Work out the finished part from the listing and answer in its coordinate system (mm). Face numbers are marked on the shaded views. A direction names the side the tool comes from. Give positions to 0.01 mm unless a question says otherwise; leave off trailing zeros. Loops run counter-clockwise (first coordinate to the right, second up) from the corner with the lowest first, then second, coordinate; pieces in that order, holes last.
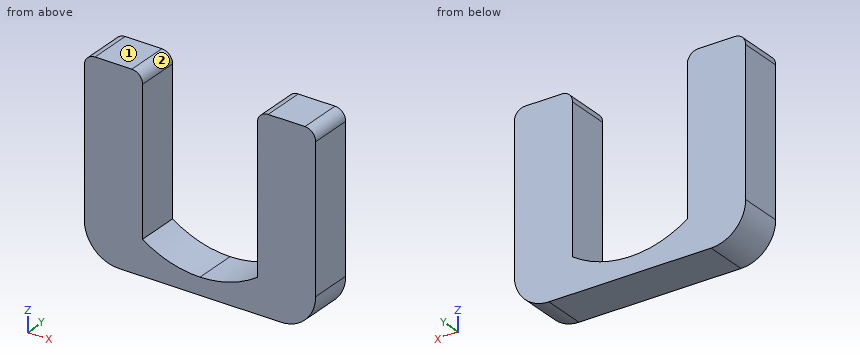
```python
from build123d import *

# Parameters (mm, degrees)
F1_DEPTH = 25.4


# Not quite as in the source:
# - the program builds the solid bodies; features that only make, move or delete a surface that nothing else refers to are left out


with BuildPart() as f1:
    # F0 (on Front) → F1 (new body)
    with BuildSketch(Plane.XZ):
        with BuildLine():
            ThreePointArc((0, -25.9232582643), (-17.7094384525, -23.2773241348), (-33.8721087757, -15.5706214843))
            Line((-33.8721087757, -15.5706214843), (-68.2603194002, -15.5706214843))
            ThreePointArc((-68.2603194002, -15.5706214843), (-62.2686711741, -30.0120658628), (-47.8133782744, -35.9702259302))
            Line((-47.8133782744, -35.9702259302), (0, -35.9702259302))
            Line((0, -35.9702259302), (47.8133782744, -35.9702259302))
            ThreePointArc((47.8133782744, -35.9702259302), (62.2686711741, -30.0120658628), (68.2603194002, -15.5706214843))
            Line((68.2603194002, -15.5706214843), (33.8721087757, -15.5706214843))
            ThreePointArc((33.8721087757, -15.5706214843), (17.7094384525, -23.2773241348), (0, -25.9232582643))
        make_face()
        with BuildLine():
            Line((-68.2603194002, -15.5706214843), (-33.8721087757, -15.5706214843))
            Line((-33.8721087757, -15.5706214843), (-33.8721087757, 69.6263722184))
            ThreePointArc((-33.8721087757, 69.6263722184), (-35.7319807152, 74.1165002789), (-40.2221087757, 75.9763722184))
            Line((-40.2221087757, 75.9763722184), (-61.9103194002, 75.9763722184))
            ThreePointArc((-61.9103194002, 75.9763722184), (-66.4004474607, 74.1165002789), (-68.2603194002, 69.6263722184))
            Line((-68.2603194002, 69.6263722184), (-68.2603194002, -15.5706214843))
        make_face()
        with BuildLine():
            Line((33.8721087757, 69.6263722184), (33.8721087757, -15.5706214843))
            Line((33.8721087757, -15.5706214843), (68.2603194002, -15.5706214843))
            Line((68.2603194002, -15.5706214843), (68.2603194002, 69.6263722184))
            ThreePointArc((68.2603194002, 69.6263722184), (66.4004474607, 74.1165002789), (61.9103194002, 75.9763722184))
            Line((61.9103194002, 75.9763722184), (40.2221087757, 75.9763722184))
            ThreePointArc((40.2221087757, 75.9763722184), (35.7319807152, 74.1165002789), (33.8721087757, 69.6263722184))
        make_face()
    extrude(amount=F1_DEPTH)


solid = f1.part
```
Q1. Section A-A on z = 35 is taken. Give the vertices of the cut face in (x, y).
Q2. Section B-B on y = -17.5 is taken. Give the vertices of the cut face in (x, z), plus the area to 3 significant figures.
Q3. Section C-C on x = 58 is taken. Give the vertices of the cut face in (y, z).
Q4. Section D-D on x = 29 is taken. Give the vertices of the cut face in (y, z).
Q5. Which of the six approach directions +Z, -Z, +X, -X, +Y, -Y give full straight-line access (tool end or side, diameter ignored) to the marked faces 1 and 2?
Q6. Given pin 1 (10 mm diameter, centred on x = 17, y = -12, fed in from +Z), flat-ended and moving along its own axis, determine where the tip first touches the part or whether it passes through.
Q7. Consider line 1 along X through (y, z) = (-8.25, 25); line 2 along X through (y, z) = (-3.75, -19); line 3 along Z through (x, y) = (-54, -3.25). Determine where each line is inside the solid, lowest interval first.
Check result:
1. outline: (-68.26, -25.4) - (-33.87, -25.4) - (-33.87, 0) - (-68.26, 0) - close; (33.87, -25.4) - (68.26, -25.4) - (68.26, 0) - (33.87, 0) - close
2. outline: (-68.26, -15.57) arc R20.4 ccw to (-47.81, -35.97) - (47.81, -35.97) arc R20.4 ccw to (68.26, -15.57) - (68.26, 69.63) arc R6.35 ccw to (61.91, 75.98) - (40.22, 75.98) arc R6.35 ccw to (33.87, 69.63) - (33.87, -15.57) arc R60.59 cw to (-33.87, -15.57) - (-33.87, 69.63) arc R6.35 ccw to (-40.22, 75.98) - (-61.91, 75.98) arc R6.35 ccw to (-68.26, 69.63) - close
2. area: 8,390 mm2
3. outline: (-25.4, -33.27) - (0, -33.27) - (0, 75.98) - (-25.4, 75.98) - close
4. outline: (-25.4, -35.97) - (0, -35.97) - (0, -18.53) - (-25.4, -18.53) - close
5. face 1: +Z, +X, -X, +Y, -Y
5. face 2: +Z, +Y, -Y
6. pin 1: stops at z = -21.79
7. line 1: x = -68.26 to -33.87, 33.87 to 68.26
7. line 2: x = -67.97 to -28.12, 28.12 to 67.97
7. line 3: z = -35.02 to 75.98
